from build123d import *

# Parameters (mm, degrees)
ESQUISSE1_R             = 1.5
EXTRUSION1_DEPTH        = 25
ESQUISSE10_W            = 8
ESQUISSE10_H            = 4
ESQUISSE10_W_2          = 7
ESQUISSE10_H_2          = 3
BOSS_EXTRU_2_DEPTH      = 0.3
ESQUISSE2_R             = 11
EXTRUSION2_DEPTH        = 2
ESQUISSE3_R             = 2.5
EXTRUSION3_DEPTH        = 17.9
ENL_V_START             = -1.6
ESQUISSE4_R             = 4
ESQUISSE4_R_2           = 2.5
ENL_V_MAT_EXTRU_1_DEPTH = 1.6
CHANFREIN1_SIZE         = 0.5
ESQUISSE6_R             = 34.95
ESQUISSE6_R_2           = 24.95
ENL_V_MAT_EXTRU_3_DEPTH = 5
ESQUISSE7_R             = 25.05
ESQUISSE7_R_2           = 19.05
ENL_V_MAT_EXTRU_4_DEPTH = 0.1
SYM_TRIE1_START         = 12.5
SYM_TRIE1_DEPTH         = 5
SYM_TRIE1_START_2       = 17.4
SYM_TRIE1_2_OUTLINE_R   = 19.05
SYM_TRIE1_2_DEPTH       = 0.1
ESQUISSE10_3_R          = 0.6
BOSS_EXTRU_3_DEPTH      = 10


# Read off the part's stored shape, not the designer's step: Symétrie1
with BuildPart() as part:
    # Esquisse1 → Extrusion1 (new body)
    with BuildSketch(Plane.XY):
        Polygon((-16.963055506, 21.15), (16.963055506, 21.15), (21.15, 16.963055506), (21.15, -16.963055506), (16.963055506, -21.15), (-16.963055506, -21.15), (-21.15, -16.963055506), (-21.15, 16.963055506), align=None)
        with Locations((-15.5, 15.5)):
            Circle(ESQUISSE1_R, mode=Mode.SUBTRACT)
        with Locations((15.5, -15.5)):
            Circle(ESQUISSE1_R, mode=Mode.SUBTRACT)
        with Locations(Location((-15.5, -15.5, 0), (0, 0, 180))):
            Circle(ESQUISSE1_R, mode=Mode.SUBTRACT)
        with Locations(Location((15.5, 15.5, 0), (0, 0, 180))):
            Circle(ESQUISSE1_R, mode=Mode.SUBTRACT)
    extrude(amount=EXTRUSION1_DEPTH)

    # Esquisse10 → Boss.-Extru.2 (add)
    with BuildSketch(Plane.XZ.offset(21.15)):
        with Locations((0, 21)):
            Rectangle(ESQUISSE10_W, ESQUISSE10_H)
        with Locations((0, 21)):
            Rectangle(ESQUISSE10_W_2, ESQUISSE10_H_2, mode=Mode.SUBTRACT)
    extrude(amount=BOSS_EXTRU_2_DEPTH)

    # Esquisse2 → Extrusion2 (add)
    with BuildSketch(Plane(origin=(0, 0, 0), x_dir=(-1, 0, 0), z_dir=(0, 0, -1))):
        with Locations(Location((0, 0, 0), (0, 0, 180))):
            Circle(ESQUISSE2_R)
    extrude(amount=EXTRUSION2_DEPTH)

    # Esquisse3 → Extrusion3 (add)
    with BuildSketch(Plane(origin=(0, 0, -2), x_dir=(-1, 0, 0), z_dir=(0, 0, -1))):
        with Locations(Location((0, 0, 0), (0, 0, 180))):
            Circle(ESQUISSE3_R)
    extrude(amount=EXTRUSION3_DEPTH)

    # Esquisse4 → Enlèv. mat.-Extru.1 (cut)
    with BuildSketch(Plane(origin=(0, 0, -2), x_dir=(-1, 0, 0), z_dir=(0, 0, -1)).offset(ENL_V_START)):
        Circle(ESQUISSE4_R)
        with Locations(Location((0, 0, 0), (0, 0, 180))):
            Circle(ESQUISSE4_R_2, mode=Mode.SUBTRACT)
    extrude(amount=ENL_V_MAT_EXTRU_1_DEPTH, mode=Mode.SUBTRACT)

    # Chanfrein1
    chanfrein1_edges = [part.edges().sort_by_distance(p)[0] for p in [
        (-2.5, 0, -19.9),
    ]]
    chamfer(chanfrein1_edges, length=CHANFREIN1_SIZE)

    # Esquisse6 → Enlèv. mat.-Extru.3 (cut)
    with BuildSketch(Plane(origin=(0, 0, 7.5), x_dir=(-1, 0, 0), z_dir=(0, 0, -1))):
        Circle(ESQUISSE6_R)
        Circle(ESQUISSE6_R_2, mode=Mode.SUBTRACT)
    extrude(amount=-ENL_V_MAT_EXTRU_3_DEPTH, mode=Mode.SUBTRACT)

    # Esquisse7 → Enlèv. mat.-Extru.4 (cut)
    with BuildSketch(Plane(origin=(0, 0, 7.5), x_dir=(-1, 0, 0), z_dir=(0, 0, -1))):
        Circle(ESQUISSE7_R)
        Circle(ESQUISSE7_R_2, mode=Mode.SUBTRACT)
    extrude(amount=-ENL_V_MAT_EXTRU_4_DEPTH, mode=Mode.SUBTRACT)

    # Symétrie1 outline → Symétrie1 (cut)
    with BuildSketch(Plane.XY.offset(SYM_TRIE1_START)):
        with BuildLine():
            Line((21.15, -16.963055506), (21.15, -13.235558167))
            ThreePointArc((21.15, -13.235558167), (17.642314191, -17.642314191), (13.235558167, -21.15))
            Line((13.235558167, -21.15), (16.963055506, -21.15))
            Line((16.963055506, -21.15), (21.15, -16.963055506))
        make_face()
        with BuildLine():
            ThreePointArc((13.235558167, 21.15), (17.642314191, 17.642314191), (21.15, 13.235558167))
            Line((21.15, 13.235558167), (21.15, 16.963055506))
            Line((21.15, 16.963055506), (16.963055506, 21.15))
            Line((16.963055506, 21.15), (13.235558167, 21.15))
        make_face()
        with BuildLine():
            Line((-16.963055506, -21.15), (-13.235558167, -21.15))
            ThreePointArc((-13.235558167, -21.15), (-17.642314191, -17.642314191), (-21.15, -13.235558167))
            Line((-21.15, -13.235558167), (-21.15, -16.963055506))
            Line((-21.15, -16.963055506), (-16.963055506, -21.15))
        make_face()
        with BuildLine():
            ThreePointArc((-21.15, 13.235558167), (-17.642314191, 17.642314191), (-13.235558167, 21.15))
            Line((-13.235558167, 21.15), (-16.963055506, 21.15))
            Line((-16.963055506, 21.15), (-21.15, 16.963055506))
            Line((-21.15, 16.963055506), (-21.15, 13.235558167))
        make_face()
    extrude(amount=SYM_TRIE1_DEPTH, mode=Mode.SUBTRACT)

    # Sym_trie1 2 outline → Sym_trie1 2 (cut)
    with BuildSketch(Plane.XY.offset(SYM_TRIE1_START_2)):
        with BuildLine():
            ThreePointArc((13.235558167, -21.15), (17.642314191, -17.642314191), (21.15, -13.235558167))
            Line((21.15, -13.235558167), (21.15, 13.235558167))
            ThreePointArc((21.15, 13.235558167), (17.642314191, 17.642314191), (13.235558167, 21.15))
            Line((13.235558167, 21.15), (-13.235558167, 21.15))
            ThreePointArc((-13.235558167, 21.15), (-17.642314191, 17.642314191), (-21.15, 13.235558167))
            Line((-21.15, 13.235558167), (-21.15, -13.235558167))
            ThreePointArc((-21.15, -13.235558167), (-17.642314191, -17.642314191), (-13.235558167, -21.15))
            Line((-13.235558167, -21.15), (13.235558167, -21.15))
        make_face()
        Circle(SYM_TRIE1_2_OUTLINE_R, mode=Mode.SUBTRACT)
    extrude(amount=SYM_TRIE1_2_DEPTH, mode=Mode.SUBTRACT)

    # Esquisse10<3> → Boss.-Extru.3 (add)
    with BuildSketch(Plane.XZ.offset(21.15)):
        with Locations(Location((2.25, 21, 0), (0, 0, 90))):
            Circle(ESQUISSE10_3_R)
        with Locations(Location((0.75, 21, 0), (0, 0, 90))):
            Circle(ESQUISSE10_3_R)
        with Locations(Location((-0.75, 21, 0), (0, 0, 90))):
            Circle(ESQUISSE10_3_R)
        with Locations(Location((-2.25, 21, 0), (0, 0, 90))):
            Circle(ESQUISSE10_3_R)
    extrude(amount=BOSS_EXTRU_3_DEPTH)


solid = part.part
The listing builds one solid part. Answer for the finished solid, in the listing's coordinates (mm). A direction names the side the tool comes from. Give positions to 0.01 mm unless a question says otherwise; leave off trailing zeros. Loops run counter-clockwise (first coordinate to the right, second up) from the corner with the lowest first, then second, coordinate; pieces in that order, holes last. Notation, with made-up numbers: (63.5, 32) - (75.5, 32) arc R23 cw to (75.5, 43) - close; hole circle Ø9 at (12, 29.25). An arc over 180 degrees is marked (long way). Answer as a JSON object with one key per item and string values.
1. Flat-ended cylindrical pins translate along their axes: pin 1 Ø1 at (y, z) = (2.5, -2) entering from +X; pin 2 Ø1 at (x, y) = (-10.5, 3) entering from -Z; pin 3 Ø3.5 at (x, y) = (-15.5, -15.5) entering from -Z. Find the tip coordinate at first contact, or state that the pin passes through.
Determined:
{"pin 1": "x = 10.82", "pin 2": "z = -2", "pin 3": "z = 0"}
2. A cutting plane is placed at A-A (z = 2.5). Write down the section's boundary in (x, y), then the cut area to 3 significant figures.
Determined:
{"outline": "(-21.15, -16.96) - (-16.96, -21.15) - (16.96, -21.15) - (21.15, -16.96) - (21.15, 16.96) - (16.96, 21.15) - (-16.96, 21.15) - (-21.15, 16.96) - close; hole circle Ø3 at (-15.5, -15.5); hole circle Ø3 at (-15.5, 15.5); hole circle Ø3 at (15.5, -15.5); hole circle Ø3 at (15.5, 15.5)", "area": "1,730 mm²"}
3. A cutting plane is placed at D-D (x = -6.5). Write down the section's boundary in (y, z).
Determined:
{"outline": "(-21.15, 0) - (-8.87, 0) - (-8.87, -2) - (8.87, -2) - (8.87, 0) - (21.15, 0) - (21.15, 7.5) - (17.91, 7.5) - (17.91, 7.6) - (21.15, 7.6) - (21.15, 17.4) - (17.91, 17.4) - (17.91, 17.5) - (21.15, 17.5) - (21.15, 25) - (-21.15, 25) - (-21.15, 17.5) - (-17.91, 17.5) - (-17.91, 17.4) - (-21.15, 17.4) - (-21.15, 7.6) - (-17.91, 7.6) - (-17.91, 7.5) - (-21.15, 7.5) - close"}
4. For faces 4 (the flat face through (0, -21.15, 21)), 5 (the flat face through (0, -21.15, 12)), 6 (the cylindrical face through (-2.38, 10.74, -0.99)), 7 (the flat face through (19.027, 19.086, 3.698)), determine the directions among +Z, -Z, +X, -X, +Y, -Y from which every point of the face is accessible in a straight line to the end or side of a thin tool.
Determined:
{"face 4": "-Y", "face 5": "-Z, +X, -X, -Y", "face 6": "-Z", "face 7": "+Z, -Z, +X, +Y"}
5. For a pull along X with two mould halves and no side action, classify faces 1 (the flat face through (0, -21.15, 4)), 2 (the flat face through (21.15, 0, 4)), 3 (the cylindrical face through (17, 15.43, 12.43)) as pulls with the +X half, pulls with the -X half, needs draft (parallel to the pull), parting line crosses it, or undercut.
Determined:
{"face 1": "needs draft", "face 2": "pulls with the +X half", "face 3": "undercut"}
6. A cutting plane is placed at B-B (y = -20). Write down the section's boundary in (x, z), then the cut area to 3 significant figures.
Determined:
{"outline": "(-18.11, 0) - (18.11, 0) - (18.11, 7.5) - (-18.11, 7.5) - close; (-18.11, 17.5) - (18.11, 17.5) - (18.11, 25) - (-18.11, 25) - close; (-14.92, 7.6) - (14.92, 7.6) - (14.92, 17.4) - (-14.92, 17.4) - close", "area": "836 mm²"}
7. Find the intervals of material crossed by L1, parallel to Y at x = -15.5, z = 19.5; L2, parallel to X at y = 15, z = 14; L3, parallel to Y at x = -15.5, z = 14.5, in increasing order. Write a range as [from, to].
Determined:
{"L1": "[-21.15, -17], [-14, 14], [17, 21.15]", "L2": "[-19.94, -16.91], [-14.09, 14.09], [16.91, 19.94]", "L3": "[-19.55, -17], [-14, 14], [17, 19.55]"}
